from build123d import *

# Parameters (mm, degrees)
F1_DEPTH = 12.7
F2_R     = 12.7
F3_DEPTH = 12.7
F4_R     = 12.7
F5_DEPTH = 25.4
F6_R     = 50.8
F7_DEPTH = 76.2
F8_R     = 38.1
F9_DEPTH = 88.9


with BuildPart() as f1:
    # F0 (on Top) → F1 (new body)
    with BuildSketch(Plane.XY):
        with BuildLine():
            Line((-115.8875, -35.319645), (-28.575, -70.639291))
            ThreePointArc((-28.575, -70.639291), (0, -76.2), (28.575, -70.639291))
            Line((28.575, -70.639291), (115.8875, -35.319645))
            ThreePointArc((115.8875, -35.319645), (139.7, 0), (115.8875, 35.319645))
            Line((115.8875, 35.319645), (28.575, 70.639291))
            ThreePointArc((28.575, 70.639291), (0, 76.2), (-28.575, 70.639291))
            Line((-28.575, 70.639291), (-115.8875, 35.319645))
            ThreePointArc((-115.8875, 35.319645), (-139.7, 0), (-115.8875, -35.319645))
        make_face()
    extrude(amount=F1_DEPTH)

    # F2 (on face) → F3 (cut, through all)
    with BuildSketch(Plane.XY.offset(12.7)):
        with Locations((-101.6, 0)):
            Circle(F2_R)
    extrude(amount=-F3_DEPTH, mode=Mode.SUBTRACT)

    # F4 (on face) → F5 (cut)
    with BuildSketch(Plane.XY.offset(12.7)):
        with Locations((101.6, 0)):
            Circle(F4_R)
    extrude(amount=-F5_DEPTH, mode=Mode.SUBTRACT)

    # F6 (on face) → F7 (join)
    with BuildSketch(Plane.XY.offset(12.7)):
        Circle(F6_R)
    extrude(amount=F7_DEPTH)

    # F8 (on face) → F9 (cut, through all)
    with BuildSketch(Plane.XY.offset(88.9)):
        Circle(F8_R)
    extrude(amount=-F9_DEPTH, mode=Mode.SUBTRACT)


solid = f1.part
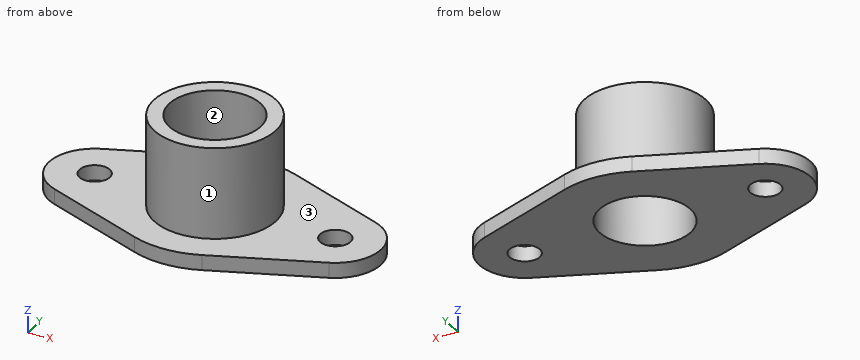
Can you work these out from the model? Positions are in its coordinate system, mm. Face numbers are marked on the shaded views. Coordinates: 2 decimals unless noted, no trailing zeros. Write each loop counter-clockwise with the first axis right and the second up, starting at its lowest first coordinate (ties: lowest second). Pieces come first, ordered by that corner, then holes. Notation, with made-up numbers: (43.25, 36.25) - (64.25, 36.25) arc R33 ccw to (64.25, 69.25) - close; hole circle Ø3 at (86, 50.5). An arc over 180 degrees is marked (long way). Return JSON: item names as keys, results as strings. Group by question number.
Item 1: If we section it at B-B (y = 0): Write out the boundary of the cut face in (x, z), then the cut area to 3 significant figures.
Item 2: Please list where these lines run through material, in increasing order: probe 1 along Z at (x, y) = (-46.5, -48); probe 2 along Y at (x, z) = (0, 55); probe 3 along Y at (x, z) = (-101, 3).
Item 3: If we section it at A-A (x = 0): Write out the boundary of the cut face in (y, z).
Item 4: We'd pull the mould along X, two halves only. Please class the marked faces 1, 2 and 3: pulls with the +X half, pulls with the -X half, needs draft (parallel to the pull), parting line crosses it, or undercut.
Item 5: If we section it at C-C (y = 19.5): Write out the boundary of the cut face in (x, z).
Item 6: I'm going to push flat-ended pins straight in: pin 1 Ø3 at (y, z) = (16, 63) entering from +X; pin 2 Ø6 at (x, y) = (61, 46) entering from +Z; pin 3 Ø8 at (x, y) = (-26.5, -28) entering from -Z; pin 4 Ø2 at (x, z) = (-60.5, 9.5) entering from +Y. Where does each tip first touch, or does it pass through?
Item 7: If we section it at D-D (z = 43.5): Write out the boundary of the cut face in (x, y), then the cut area to 3 significant figures.
Return value:
{
 "1": {"outline": "(-139.7, 0) - (-114.3, 0) - (-114.3, 12.7) - (-139.7, 12.7) - close; (-88.9, 0) - (-38.1, 0) - (-38.1, 88.9) - (-50.8, 88.9) - (-50.8, 12.7) - (-88.9, 12.7) - close; (38.1, 0) - (88.9, 0) - (88.9, 12.7) - (50.8, 12.7) - (50.8, 88.9) - (38.1, 88.9) - close; (114.3, 0) - (139.7, 0) - (139.7, 12.7) - (114.3, 12.7) - close", "area": "3,870 mm^2"},
 "2": {"probe 1": "z = 0 to 12.7", "probe 2": "y = -50.8 to -38.1, 38.1 to 50.8", "probe 3": "y = -41.34 to -12.69, 12.69 to 41.34"},
 "3": {"outline": "(-76.2, 0) - (-38.1, 0) - (-38.1, 88.9) - (-50.8, 88.9) - (-50.8, 12.7) - (-76.2, 12.7) - close; (38.1, 0) - (76.2, 0) - (76.2, 12.7) - (50.8, 12.7) - (50.8, 88.9) - (38.1, 88.9) - close"},
 "4": {"face 1": "parting line crosses it", "face 2": "undercut", "face 3": "needs draft"},
 "5": {"outline": "(-134.33, 0) - (-32.73, 0) - (-32.73, 88.9) - (-46.91, 88.9) - (-46.91, 12.7) - (-134.33, 12.7) - close; (32.73, 0) - (134.33, 0) - (134.33, 12.7) - (46.91, 12.7) - (46.91, 88.9) - (32.73, 88.9) - close"},
 "6": {"pin 1": "stops at x = 48.69", "pin 2": "stops at z = 12.7", "pin 3": "stops at z = 0", "pin 4": "stops at y = 58.13"},
 "7": {"outline": "circle Ø101.6 at (0, 0); hole circle Ø76.2 at (0, 0)", "area": "3,550 mm^2"}
}
